Source: CAD feature listing. Evaluate the final solid. Frame: model axes, mm. Give positions to 0.01 mm unless a question says otherwise; leave off trailing zeros. Order: outer loops, then holes, each group sorted by start corner. A loop starts at its lowest first (then second) coordinate and runs counter-clockwise, first axis right, second up.
Autodesk Inventor part; units mm, degrees
ref_plane "YZ Plane" through (0, 0, 0) normal (1, 0, 0) x (0, 1, 0)
ref_plane "XZ Plane" through (0, 0, 0) normal (0, 1, 0) x (-1, 0, 0)
ref_plane "XY Plane" through (0, 0, 0) normal (0, 0, 1) x (1, 0, 0)
sketch "スケッチ1" plane through (0, 0, 0) normal (0, 0, 1) x (1, 0, 0)
  line L0 (-25, 25) -> (25, 25)
  line L1 (25, 25) -> (25, -25)
  line L2 (25, -25) -> (-25, -25)
  line L3 (-25, -25) -> (-25, 25)
  line L4 (-23, 23) -> (23, 23)
  line L5 (23, 23) -> (23, -23)
  line L6 (23, -23) -> (-23, -23)
  line L7 (-23, -23) -> (-23, 23)
  point P0 (0, 0)
  dimension "d0" = 50
  dimension "d1" = 50
  dimension "d4" = 25
  dimension "d5" = 25
  dimension "d6" = 46
  dimension "d7" = 2
  dimension "d8" = 46
  dimension "d9" = 2
extrude "押し出し1" add sketch "スケッチ1" along normal blind 50
sketch "スケッチ11" plane through (25, -25, 0) normal (1, 0, 0) x (0, 0, -1)
  circle A0 centre (-36.5, 36.5) radius 1.5
  line L0 (-50, 50) -> (-50, 0)
  circle A1 centre (-27.5, 12.5) radius 1.5
  line L1 (0, 50) -> (0, 0)
  line L2 (0, 50) -> (-50, 50)
  point P0 (0, 25)
  point P1 (-50, 43)
  dimension "d192" = 118
  dimension "d109" = 3
  dimension "d128" = 24
  dimension "d237" = 13.5
  dimension "d238" = 27.5
  dimension "d239" = 13.5
hole "穴6" at (25, -12.5, 27.5) at (25, 11.5, 36.5) direction (-1, 0, 0) diameter 4 end through all
sketch "スケッチ15" plane through (-25, -25, 0) normal (0, -1, 0) x (1, 0, 0)
  line L0 (50, 50) -> (0, 50)
  line L1 (0, 0) -> (0, 50)
  circle A0 centre (10, 47.75) radius 1
  circle A1 centre (25, 47.75) radius 1
  circle A2 centre (40, 47.75) radius 1
  line L2 (50, 0) -> (0, 0)
  circle A3 centre (10, 2.25) radius 1
  circle A4 centre (25, 2.25) radius 1
  circle A5 centre (40, 2.25) radius 1
  point P0 (49.5, 0)
  point P1 (49.5, 50)
  point P2 (25, 0)
  dimension "d138" = 2
  dimension "d139" = 10
  dimension "d141" = 2.25
  dimension "d142" = 2.25
  dimension "d143" = 2.25
  dimension "d144" = 15
  dimension "d166" = 15
  dimension "d167" = 10
  dimension "d168" = 15
  dimension "d169" = 15
  dimension "d170" = 2.25
  dimension "d171" = 2.25
  dimension "d172" = 2.25
hole "穴10" at (-15, -25, 47.75) at (-15, -25, 2.25) at (0, -25, 47.75) at (0, -25, 2.25) at (15, -25, 2.25) at (15, -25, 47.75) direction (0, 1, 0) diameter 2 end through all
sketch "スケッチ16" plane through (-25, -25, 0) normal (-1, 0, 0) x (0, 0, 1)
  line L0 (50, 0) -> (50, 50)
  line L1 (0, 50) -> (50, 50)
  line L2 (0, 0) -> (50, 0)
  circle A0 centre (47.75, 40) radius 1
  circle A1 centre (47.75, 25) radius 1
  circle A2 centre (47.75, 10) radius 1
  circle A3 centre (2.25, 40) radius 1
  circle A4 centre (2.25, 25) radius 1
  circle A5 centre (2.25, 10) radius 1
  line L3 (0, 48) -> (0, 2)
  point P0 (0, 25)
  dimension "d152" = 2
  dimension "d153" = 2.25
  dimension "d154" = 2.25
  dimension "d155" = 2.25
  dimension "d156" = 10
  dimension "d157" = 10
  dimension "d158" = 15
  dimension "d173" = 15
  dimension "d174" = 15
  dimension "d175" = 10
  dimension "d176" = 2.25
  dimension "d177" = 2.25
  dimension "d178" = 2.25
hole "穴11" at (-25, 15, 2.25) at (-25, 0, 2.25) at (-25, -15, 2.25) at (-25, -15, 47.75) at (-25, 0, 47.75) at (-25, 15, 47.75) direction (1, 0, 0) diameter 2 end through all
sketch "スケッチ18" plane through (-25, -25, 0) normal (0, -1, 0) x (1, 0, 0)
  circle A0 centre (25, 2.25) radius 1
  circle A1 centre (25, 47.75) radius 1
  line L0 (50, 50) -> (0, 50)
  line L1 (50, 0) -> (0, 0)
  circle A2 centre (14, 40) radius 1.5
  circle A3 centre (36, 40) radius 1.5
  circle A4 centre (14, 10) radius 1.5
  circle A5 centre (36, 10) radius 1.5
  point P0 (49.5, 0)
  point P1 (49.5, 50)
  point P2 (25, 0)
  dimension "d240" = 10
  dimension "d241" = 10
  dimension "d242" = 10
  dimension "d243" = 10
  dimension "d244" = 11
  dimension "d245" = 11
  dimension "d246" = 11
  dimension "d247" = 11
  dimension "d248" = 3
hole "穴13" at (-11, -25, 40) at (-11, -25, 10) at (11, -25, 40) at (11, -25, 10) direction (0, 1, 0) diameter 3 depth 2 tip angle 118
thread "ねじ13"
thread "ねじ14"
thread "ねじ15"
thread "ねじ16"
1) Pin query (flat end, axial travel): pin 1 (1.8 mm diameter, centred on y = 15, z = 2.25, fed in from +X). Return the tip coordinate at first contact, or that it passes through.
Report:
pin 1: passes through
2) Section query A-A, the plane z = 40. Return the cut outline in (x, y), and give its area (3 significant figures).
Report:
outline: (-25, -25) - (-12.5, -25) - (-12.5, -23) - (-23, -23) - (-23, 23) - (23, 23) - (23, -23) - (12.5, -23) - (12.5, -25) - (25, -25) - (25, 25) - (-25, 25) - close; (-9.5, -25) - (9.5, -25) - (9.5, -23) - (-9.5, -23) - close
area: 372 mm2
3) Section query D-D, the plane x = -11. Return the cut outline in (y, z), and give its area (3 significant figures).
Report:
outline: (-25, 0) - (-23, 0) - (-23, 8.5) - (-25, 8.5) - close; (-25, 11.5) - (-23, 11.5) - (-23, 38.5) - (-25, 38.5) - close; (-25, 41.5) - (-23, 41.5) - (-23, 50) - (-25, 50) - close; (23, 0) - (25, 0) - (25, 50) - (23, 50) - close
area: 188 mm2
4) Material intervals for L1, parallel to X at y = 1.5, z = 10.5; L2, parallel to Z at x = 0, y = 23.95, sorted ascending.
Report:
L1: x = -25 to -23, 23 to 25
L2: z = 0 to 1.25, 3.25 to 46.75, 48.75 to 50
5) Draft query along Z for faces 1 (the cylindrical face through (-23.986, -14.024, 2.033)), 2 (the flat face through (0, -25, 25)), 3 (the flat face through (-2, -24, 0)). Return one class per face: +Z half, -Z half, draft (parallel to the pull), parting line (faces both ways), or undercut.
Report:
face 1: undercut
face 2: draft
face 3: -Z half
6) Section query B-B, the plane y = -7.5. Return the cut outline in (x, z), and give its area (3 significant figures).
Report:
outline: (-25, 0) - (-23, 0) - (-23, 50) - (-25, 50) - close; (23, 0) - (25, 0) - (25, 50) - (23, 50) - close
area: 200 mm2
